```python
from build123d import *

# Parameters (mm, degrees)
SKETCH1_R           = 8.5
BOSS_EXTRUDE1_DEPTH = 40
BOSS_EXTRUDE2_START = -8
SKETCH2_W           = 6
SKETCH2_H           = 6
BOSS_EXTRUDE2_DEPTH = 8
SKETCH3_OUTSIDE_W   = 43.662
SKETCH3_OUTSIDE_H   = 43.662
CUT_EXTRUDE1_DEPTH  = 6
FILLET2_R           = 0.6


with BuildPart() as part:
    # Sketch1 → Boss-Extrude1 (new body)
    with BuildSketch(Plane.XY):
        Circle(SKETCH1_R)
    extrude(amount=BOSS_EXTRUDE1_DEPTH)

    # Sketch2 → Boss-Extrude2 (add)
    with BuildSketch(Plane.XY.offset(40).offset(BOSS_EXTRUDE2_START)):
        with BuildLine():
            Line((3, 7.95298686), (3, 15))
            Line((3, 15), (-3, 15))
            Line((-3, 15), (-3, 7.95298686))
            ThreePointArc((-3, 7.95298686), (0, 8.5), (3, 7.95298686))
        make_face()
        with BuildLine():
            Line((-7.95298686, 3), (-3, 3))
            Line((-3, 3), (-3, 7.95298686))
            ThreePointArc((-3, 7.95298686), (-6.01040764, 6.01040764), (-7.95298686, 3))
        make_face()
        with BuildLine():
            Line((-3, 7.95298686), (-3, 15))
            ThreePointArc((-3, 15), (-6.514718626, 6.514718626), (-15, 3))
            Line((-15, 3), (-7.95298686, 3))
            ThreePointArc((-7.95298686, 3), (-6.01040764, 6.01040764), (-3, 7.95298686))
        make_face()
        with BuildLine():
            Line((-3, 3), (3, 3))
            Line((3, 3), (3, 7.95298686))
            ThreePointArc((3, 7.95298686), (0, 8.5), (-3, 7.95298686))
            Line((-3, 7.95298686), (-3, 3))
        make_face()
        Rectangle(SKETCH2_W, SKETCH2_H)
        with BuildLine():
            Line((-3, -3), (-3, 3))
            Line((-3, 3), (-7.95298686, 3))
            ThreePointArc((-7.95298686, 3), (-8.5, 0), (-7.95298686, -3))
            Line((-7.95298686, -3), (-3, -3))
        make_face()
        with BuildLine():
            Line((-7.95298686, 3), (-15, 3))
            Line((-15, 3), (-15, -3))
            Line((-15, -3), (-7.95298686, -3))
            ThreePointArc((-7.95298686, -3), (-8.5, 0), (-7.95298686, 3))
        make_face()
        with BuildLine():
            ThreePointArc((-15, -3), (-6.514718626, -6.514718626), (-3, -15))
            Line((-3, -15), (-3, -7.95298686))
            ThreePointArc((-3, -7.95298686), (-6.01040764, -6.01040764), (-7.95298686, -3))
            Line((-7.95298686, -3), (-15, -3))
        make_face()
        with BuildLine():
            Line((-3, -7.95298686), (-3, -3))
            Line((-3, -3), (-7.95298686, -3))
            ThreePointArc((-7.95298686, -3), (-6.01040764, -6.01040764), (-3, -7.95298686))
        make_face()
        with BuildLine():
            Line((3, -7.95298686), (3, -3))
            Line((3, -3), (-3, -3))
            Line((-3, -3), (-3, -7.95298686))
            ThreePointArc((-3, -7.95298686), (0, -8.5), (3, -7.95298686))
        make_face()
        with BuildLine():
            ThreePointArc((3, -7.95298686), (6.01040764, -6.01040764), (7.95298686, -3))
            Line((7.95298686, -3), (3, -3))
            Line((3, -3), (3, -7.95298686))
        make_face()
        with BuildLine():
            ThreePointArc((8.5, 0), (8.362128566, 1.524731401), (7.95298686, 3))
            Line((7.95298686, 3), (3, 3))
            Line((3, 3), (3, -3))
            Line((3, -3), (7.95298686, -3))
            ThreePointArc((7.95298686, -3), (8.362128566, -1.524731401), (8.5, 0))
        make_face()
        with BuildLine():
            ThreePointArc((3, -15), (6.514718626, -6.514718626), (15, -3))
            Line((15, -3), (7.95298686, -3))
            ThreePointArc((7.95298686, -3), (6.01040764, -6.01040764), (3, -7.95298686))
            Line((3, -7.95298686), (3, -15))
        make_face()
        with BuildLine():
            Line((15, -3), (15, 3))
            Line((15, 3), (7.95298686, 3))
            ThreePointArc((7.95298686, 3), (8.362128566, 1.524731401), (8.5, 0))
            ThreePointArc((8.5, 0), (8.362128566, -1.524731401), (7.95298686, -3))
            Line((7.95298686, -3), (15, -3))
        make_face()
        with BuildLine():
            Line((7.95298686, 3), (15, 3))
            ThreePointArc((15, 3), (6.514718626, 6.514718626), (3, 15))
            Line((3, 15), (3, 7.95298686))
            ThreePointArc((3, 7.95298686), (6.01040764, 6.01040764), (7.95298686, 3))
        make_face()
        with BuildLine():
            Line((3, 3), (7.95298686, 3))
            ThreePointArc((7.95298686, 3), (6.01040764, 6.01040764), (3, 7.95298686))
            Line((3, 7.95298686), (3, 3))
        make_face()
        with BuildLine():
            Line((-3, -15), (3, -15))
            Line((3, -15), (3, -7.95298686))
            ThreePointArc((3, -7.95298686), (0, -8.5), (-3, -7.95298686))
            Line((-3, -7.95298686), (-3, -15))
        make_face()
    extrude(amount=BOSS_EXTRUDE2_DEPTH)

    # Sketch3 outside → Cut-Extrude1 (cut)
    with BuildSketch(Plane(origin=(0, 0, 0), x_dir=(-1, 0, 0), z_dir=(0, 0, -1))):
        Rectangle(SKETCH3_OUTSIDE_W, SKETCH3_OUTSIDE_H)
        Polygon((4.25, 7.361215932), (-4.25, 7.361215932), (-8.5, 0), (-4.25, -7.361215932), (4.25, -7.361215932), (8.5, 0), align=None, mode=Mode.SUBTRACT)
    extrude(amount=-CUT_EXTRUDE1_DEPTH, mode=Mode.SUBTRACT)

    # Fillet2
    fillet2_edges = [part.edges().sort_by_distance(p)[0] for p in [
        (15, 0, 32),
        (6.514718626, -6.514718626, 32),
        (0, -15, 32),
        (0, 15, 40),
        (-6.514718626, 6.514718626, 40),
        (-15, 0, 40),
        (-6.514718626, -6.514718626, 40),
        (-3, -15, 36),
        (-15, 0, 32),
        (-15, -3, 36),
        (-6.514718626, 6.514718626, 32),
        (-15, 3, 36),
        (0, 15, 32),
        (-3, 15, 36),
        (6.514718626, 6.514718626, 40),
        (3, 15, 36),
        (15, 0, 40),
        (15, 3, 36),
        (6.514718626, -6.514718626, 40),
        (15, -3, 36),
        (0, -15, 40),
        (3, -15, 36),
        (-6.514718626, -6.514718626, 32),
        (6.514718626, 6.514718626, 32),
    ]]
    fillet(fillet2_edges, radius=FILLET2_R)


solid = part.part
```
Check sheet for the modelled part. Datum: model origin and axes. Units: mm. A direction names the side the tool comes from. Round coordinates to 2 decimals unless told otherwise and drop trailing zeros. Loops run counter-clockwise (first coordinate to the right, second up) from the corner with the lowest first, then second, coordinate; pieces in that order, holes last. Notation, with made-up numbers: (-17, -25.5) - (29, -25.5) arc R12 cw to (29, -12.5) - close; hole circle Ø7 at (17, -12.5). An arc over 180 degrees is marked (long way). Answer as a JSON object with one key per item and string values. Group by question number.
Q1. Scan lines: line 1 along Z through (x, y) = (-2.25, 9.25); line 2 along Z through (x, y) = (1.25, -7.5); line 3 along X through (y, z) = (-5.25, 17.5). Record each from-to range of solid material in increasing order. Write a range as [from, to].
Q2. Sectioned sample at B-B, the plane z = 20. Enter the section's corners in (x, y).
Q3. Gauge pin test, flat ends, axial feed: P1, Ø2, axis at x = 7.5, y = -3, coming from the -Z side; P2, Ø4, axis at x = 2, z = 12.5, coming from the -Y side; P3, Ø2, axis at y = -3, z = 12, coming from the +X side; P4, Ø1.5, axis at x = -5, z = 8.5, coming from the -Y side. Record the tip position at first contact, or that the pin passes through.
Q4. Sectioned sample at A-A, the plane x = 0. Enter the section's corners in (y, z), plus the area to 3 significant figures.
Q5. Set-up check for faces 1 (the face through (0, 7.361, 3)), 2 (the face through (0, -8, 6)), 3 (the face through (-7, -4, 6)), 4 (the face through (4.57, 7.167, 18.818)), 5 (the face through (-6.405, 3.629, 2.958)): record each of +Z, -Z, +X, -X, +Y, -Y from which the full face is reachable in a straight line by a thin tool's end or side.
Solution:
{
 "1": {"line 1": "z = [32, 40]", "line 2": "z = [6, 40]", "line 3": "x = [-6.68, 6.68]"},
 "2": {"outline": "circle Ø17 at (0, 0)"},
 "3": {"P1": "stops at z = 0", "P2": "stops at y = -8.5", "P3": "stops at x = 8.26", "P4": "stops at y = -7.36"},
 "4": {"outline": "(-15, 32.6) arc R0.6 ccw to (-14.4, 32) - (-8.5, 32) - (-8.5, 6) - (-7.36, 6) - (-7.36, 0) - (7.36, 0) - (7.36, 6) - (8.5, 6) - (8.5, 32) - (14.4, 32) arc R0.6 ccw to (15, 32.6) - (15, 39.4) arc R0.6 ccw to (14.4, 40) - (-14.4, 40) arc R0.6 ccw to (-15, 39.4) - close", "area": "770 mm²"},
 "5": {"face 1": "-Z, +X, -X, +Y", "face 2": "-Z, +X, -X, -Y", "face 3": "-Z, -X, -Y", "face 4": "-Z", "face 5": "-Z, -X, +Y"}
}
